Autodesk Inventor part; units mm, degrees
ref_plane "YZ Plane" through (0, 0, 0) normal (1, 0, 0) x (0, 1, 0)
ref_plane "XZ Plane" through (0, 0, 0) normal (0, 1, 0) x (-1, 0, 0)
ref_plane "XY Plane" through (0, 0, 0) normal (0, 0, 1) x (1, 0, 0)
sketch "Sketch1" plane through (0, 0, 0) normal (0, 0, 1) x (1, 0, 0)
  line L0 (-60, 60) -> (60, 60)
  line L1 (60, 60) -> (60, -60)
  line L2 (60, -60) -> (-60, -60)
  line L3 (-60, -60) -> (-60, 60)
  line L4 (-60, 60) -> (60, -60) construction
  line L5 (60, 60) -> (-60, -60) construction
  point P0 (0, 0)
  dimension "d0" = 120
  dimension "d1" = 120
extrude "Extrusion1" add sketch "Sketch1" along normal blind 1000
sketch "Sketch2" plane through (0, 0, 1000) normal (0, 0, 1) x (1, 0, 0)
  line L0 (-50, 50) -> (50, 50)
  line L1 (50, 50) -> (50, -50)
  line L2 (50, -50) -> (-50, -50)
  line L3 (-50, -50) -> (-50, 50)
  line L4 (-50, 50) -> (50, -50) construction
  line L5 (50, 50) -> (-50, -50) construction
  point P0 (0, 0)
  dimension "d4" = 100
  dimension "d5" = 100
extrude "Extrusion2" cut sketch "Sketch2" against normal blind 1000
sketch "Sketch3" plane through (60, -60, 0) normal (1, 0, 0) x (0, 0, -1)
  line L0 (0, 0) -> (-1000, 0)
  line L1 (-1072.8828, 120) -> (-1072.8828, 60)
  line L2 (-1072.8828, 60) -> (45.9524, 60)
  circle A0 centre (-800, 60) radius 25
  line L3 (-1000, 120) -> (-1072.8828, 120)
  line L4 (-1000, 120) -> (-1000, 166.4974)
  line L5 (-800, 60) -> (-800, 166.4974)
  line L6 (-650, 60) -> (-650, 175.0662)
  line L7 (-500, 60) -> (-500, 175.0662)
  circle A1 centre (-650, 60) radius 25
  circle A2 centre (-500, 60) radius 25
  line L8 (-350, 60) -> (-350, 191.0617)
  circle A3 centre (-350, 60) radius 25
  point P0 (0, 60)
  dimension "d9" = 50
  dimension "d10" = 60
  dimension "d12" = 200
  dimension "d13" = 150
  dimension "d14" = 150
  dimension "d15" = 50
  dimension "d16" = 50
  dimension "d17" = 150
  dimension "d18" = 50
extrude "Extrusion3" cut sketch "Sketch3" against normal blind 1000
sketch "Sketch4" plane through (60, -60, 0) normal (1, 0, 0) x (0, 0, -1)
  line L0 (0, 0) -> (-1000, 0)
  line L1 (-1000, -138.0957) -> (-425, -138.0957)
  line L2 (-425, -90) -> (-500, 0)
  line L3 (-425, -90) -> (-350, 0)
  point P0 (0, 60)
  dimension "d21" = 575
extrude "Extrusion4" add sketch "Sketch4" against normal blind 120
fillet "Fillet1" radius 30 1 edges at (0, -150, 425)
sketch "Sketch5" plane through (60, -60, 0) normal (1, 0, 0) x (0, 0, -1)
  line L0 (-500, 0) -> (-1000, 0)
  circle A0 centre (-425, -30) radius 17.5
  line L1 (-425, -6.2892) -> (-425, -12.5)
  point P0 (0, 60)
extrude "Extrusion5" cut sketch "Sketch5" against normal blind 120
sketch "Sketch11" plane through (0, 0, 0) normal (1, 0, 0) x (0, 1, 0)
  line L0 (0, 0) -> (-191.3129, 0)
  line L1 (-191.3129, 0) -> (-191.3129, 1000)
  line L2 (-340.1694, 1000) -> (-340.1694, 500)
  line L3 (-340.1694, 500) -> (94.4413, 500)
  line L4 (-60.9651, 500) -> (-60.9651, 425)
  line L5 (-150.9651, 425) -> (-60.9651, 500)
  line L6 (-60.9651, 425) -> (-60.9651, 350)
  line L7 (-60.9651, 350) -> (-150.9651, 425)
  dimension "d33" = 1000
  dimension "d35" = 500
extrude "Extrusion6" cut sketch "Sketch11" along normal mid plane 100
sketch "Sketch12" plane through (60, -60, 0) normal (1, 0, 0) x (0, 0, -1)
  circle A0 centre (-100, 60) radius 10
  circle A1 centre (-140, 60) radius 10
  circle A2 centre (-180, 60) radius 10
  point P0 (0, 60)
  dimension "d41" = 20
  dimension "d42" = 20
  dimension "d43" = 20
  dimension "d44" = 40
  dimension "d45" = 40
  dimension "d46" = 100
extrude "Extrusion7" cut sketch "Sketch12" against normal blind 599.25
properties part number "atas 1"
Design review of the part built by this model. Coordinates are the model's own, in mm. A direction names the side the tool comes from. Give positions to 0.01 mm unless a question says otherwise; leave off trailing zeros. Loops run counter-clockwise (first coordinate to the right, second up) from the corner with the lowest first, then second, coordinate; pieces in that order, holes last. Notation, with made-up numbers: (72, -26) -> (76, -26) arc R19 cw to (76, -15) -> close; hole circle Ø2 at (80, 44). An arc over 180 degrees is marked (long way). One line per question, with ' | ' between items. Start each with the question number.
(1) We need section C-C (x = 35). State the section outline as (y, z) points, and give its area (3 significant figures).
(2) Insertion check: P1, Ø1.5, axis at x = -6.5, z = 205.5, coming from the -Y side; P2, Ø2, axis at x = -17.5, z = 435.5, coming from the -Y side. Each pin has a flat end and moves straight along its axis. Give the tip position at first contact, or say it passes through.
(3) For line 1 (Y direction, x = -45.5, z = 727); line 2 (Y direction, x = -54.5, z = 800), list the stretches that pass through material, from the lowest coordinate up.
(4) We need section A-A (z = 425). State the section outline as (x, y) points.
(5) We need section B-B (y = -90). State the section outline as (x, z) points, and give its area (3 significant figures).
(6) Draft analysis for pull direction X (two halves, no side actions). For faces 1 (the face through (-1, 50, 507)), 2 (the face through (60, -35, 493)), 3 (the face through (-53.1, -93.6, 472)), state which applies: +X half, -X half, draft (parallel to the pull), parting line (faces both ways), or undercut.
(7) For faces 4 (the face through (55.07, 7.509, 626.154)), 5 (the face through (1, -50, 507)), 6 (the face through (-50, -90, 443)), list the 3-axis set-ups (+Z, -Z, +X, -X, +Y, -Y) from which the entire face can be reached by the end or side of a thin tool; tool diameter is ignored.
(8) We need section D-D (z = 200). State the section outline as (x, y) points, and give its area (3 significant figures).
The answers:
1) outline: (-60.97, 350.8) -> (-60, 350) -> (-60, 0) -> (-50, 0) -> (-50, 1000) -> (-60, 1000) -> (-60, 500) -> (-60.97, 499.2) -> close; (50, 0) -> (60, 0) -> (60, 1000) -> (50, 1000) -> close | area: 20,100 mm^2
2) P1: stops at y = -60 | P2: stops at y = -60.97
3) line 1: y = -60 to -50, 50 to 60 | line 2: y = -60 to -25, 25 to 60
4) outline: (-60, -133.14) -> (-50, -133.14) -> (-50, -107.5) -> (-60, -107.5) -> close; (-60, -72.5) -> (-50, -72.5) -> (-50, -60.97) -> (50, -60.97) -> (50, -72.5) -> (60, -72.5) -> (60, 60) -> (-60, 60) -> close; (50, -133.14) -> (60, -133.14) -> (60, -107.5) -> (50, -107.5) -> close; hole (-50, -50) -> (50, -50) -> (50, 50) -> (-50, 50) -> close
5) outline: (-60, 375) -> (-50, 375) -> (-50, 407.5) -> (-60, 407.5) -> close; (-60, 442.5) -> (-50, 442.5) -> (-50, 475) -> (-60, 475) -> close; (50, 375) -> (60, 375) -> (60, 407.5) -> (50, 407.5) -> close; (50, 442.5) -> (60, 442.5) -> (60, 475) -> (50, 475) -> close | area: 1,300 mm^2
6) face 1: undercut | face 2: +X half | face 3: draft
7) face 4: +X, -X | face 5: +Z, -Z | face 6: +Z, -Z, -Y
8) outline: (-60, -60) -> (60, -60) -> (60, 60) -> (-60, 60) -> close; hole (-50, -50) -> (50, -50) -> (50, 50) -> (-50, 50) -> close | area: 4,400 mm^2
